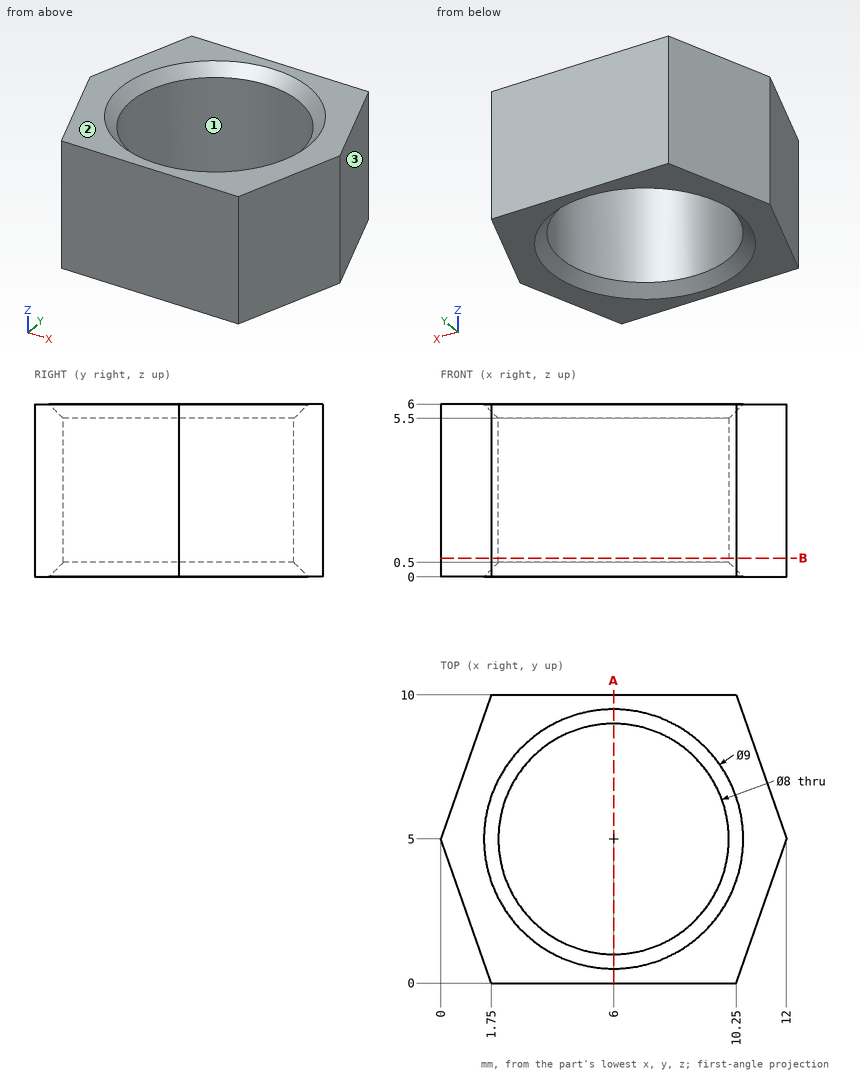
Source: three-view drawing plus pictorial views. Frame: mm from the lowest corner of the part. Coordinates: 2 decimals unless noted, no trailing zeros. Loops run counter-clockwise (first coordinate to the right, second up) from the corner with the lowest first, then second, coordinate; pieces in that order, holes last. Notation, with made-up numbers: (28, 82) - (64, 82) arc R23 ccw to (64, 93) - close; hole circle Ø10 at (51, -34.75). An arc over 180 degrees is marked (long way). One line per item, written item: value. Start each with the question number.
1. Ray query, L1, parallel to Y at x = 6, z = 4.1; L2, parallel to Y at x = 3, z = 4.6; L3, parallel to X at y = 1.75, z = 1.65. Return the intervals inside material, ascending.
2. Section B-B (z = 0.65). Return the cut outline in (x, y).
3. Mould query, pull axis Y, two halves, no side actions, for the marked faces 1, 2 and 3. Classes: pulls with the +Y half, pulls with the -Y half, needs draft (parallel to the pull), parting line crosses it, or undercut.
4. Section A-A (x = 6). Return the cut outline in (y, z), and give its area (3 significant figures).
5. Contact query for a flat-ended pin moving along its axis: P1, Ø3, axis at y = 9, z = 4.5, coming from the +X side (3 decimals). Output: stop coordinate, or through.
Verdict:
1. L1: y = 0 to 1, 9 to 10
1. L2: y = 0 to 2.35, 7.65 to 10
1. L3: x = 1.14 to 3.67, 8.33 to 10.86
2. outline: (0, 5) - (1.75, 0) - (10.25, 0) - (12, 5) - (10.25, 10) - (1.75, 10) - close; hole circle Ø8 at (6, 5)
3. face 1: undercut
3. face 2: needs draft
3. face 3: pulls with the +Y half
4. outline: (0, 0) - (0.5, 0) - (1, 0.5) - (1, 5.5) - (0.5, 6) - (0, 6) - close; (9, 0.5) - (9.5, 0) - (10, 0) - (10, 6) - (9.5, 6) - (9, 5.5) - close
4. area: 11.5 mm2
5. P1: stops at x = 11.125
